from build123d import *

# Parameters (mm, degrees)
SKETCH1_R           = 5.715
BOSS_EXTRUDE1_DEPTH = 12.7
SKETCH2_R           = 1.4732
CUT_EXTRUDE1_DEPTH  = 16.053652381
SKETCH3_W           = 7
SKETCH3_H           = 6
BOSS_EXTRUDE2_DEPTH = 7


with BuildPart() as part:
    # Sketch1 → Boss-Extrude1 (new body)
    with BuildSketch(Plane.XY):
        with Locations(Location((0, 0, 0), (0, 0, 180))):
            Circle(SKETCH1_R)
    extrude(amount=BOSS_EXTRUDE1_DEPTH)

    # Sketch2 → Cut-Extrude1 (cut, through all)
    with BuildSketch(Plane.XY.offset(12.7)):
        Circle(SKETCH2_R)
    extrude(amount=-CUT_EXTRUDE1_DEPTH, mode=Mode.SUBTRACT)

    # Sketch3 → Boss-Extrude2 (add)
    with BuildSketch(Plane(origin=(4, 0, 0), x_dir=(0, 0, -1), z_dir=(1, 0, 0))):
        with Locations((-6.35, 0)):
            Rectangle(SKETCH3_W, SKETCH3_H)
    extrude(amount=BOSS_EXTRUDE2_DEPTH)


solid = part.part
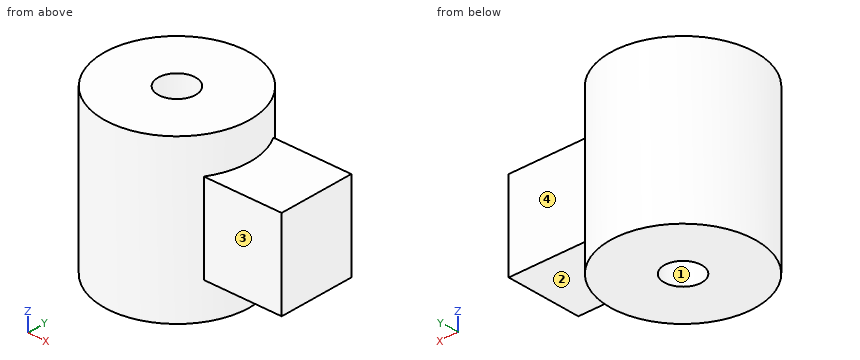
Read the model definition and answer for the solid it produces. Units are mm, in the model's axes. Face numbers are marked on the shaded views. Give positions to 0.01 mm unless a question says otherwise; leave off trailing zeros. Write each loop counter-clockwise with the first axis right and the second up, starting at its lowest first coordinate (ties: lowest second). Pieces come first, ordered by that corner, then holes. Notation, with made-up numbers: (-36, 11.5) -> (-13, 11.5) arc R30 cw to (-13, 40.5) -> close; hole circle Ø11 at (-29, 15). An arc over 180 degrees is marked (long way). Answer as a JSON object with one key per item and string values. Group by question number.
1) Consider L1, parallel to Y at x = 0, z = 5 (3 decimals); L2, parallel to Y at x = 7.25, z = 8; L3, parallel to Z at x = 9.5, y = -0.5. Determine where each line is inside the solid, lowest interval first. Write a range as from..to.
2) Each of these flat-tipped pins is pushed along its axis until it touches: P1, Ø4, axis at x = 7, z = 4.5, coming from the -Y side; P2, Ø6.5, axis at x = 8.5, z = 6, coming from the +Y side; P3, Ø3, axis at x = 8, y = -0.5, coming from the -Z side. Where does it stop, or does it pass through?
3) The mould has two halves that part along Y. Classify the marked faces 1, 2, 3 and 4: +Y half, -Y half, draft (parallel to the pull), parting line (faces both ways), or undercut.
4) Find section A-A (x = 0). Write down the section's boundary in (y, z) (3 decimals).
5) Find section D-D (y = 2.5). Write down the section's boundary in (x, z), and give its area (3 significant figures).
6) Find section C-C (z = 10.5). Write down the section's boundary in (x, y) (3 decimals).
7) Find section B-B (y = 0). Write down the section's boundary in (x, z) (3 decimals), and give its area (3 significant figures).
Values follow:
{
 "1": {"L1": "y = -5.715..-1.473, 1.473..5.715", "L2": "y = -3..3", "L3": "z = 2.85..9.85"},
 "2": {"P1": "stops at y = -3", "P2": "stops at y = 3", "P3": "stops at z = 2.85"},
 "3": {"face 1": "undercut", "face 2": "draft", "face 3": "-Y half", "face 4": "+Y half"},
 "4": {"outline": "(-5.715, 0) -> (-1.473, 0) -> (-1.473, 12.7) -> (-5.715, 12.7) -> close; (1.473, 0) -> (5.715, 0) -> (5.715, 12.7) -> (1.473, 12.7) -> close"},
 "5": {"outline": "(-5.14, 0) -> (5.14, 0) -> (5.14, 2.85) -> (11, 2.85) -> (11, 9.85) -> (5.14, 9.85) -> (5.14, 12.7) -> (-5.14, 12.7) -> close", "area": "172 mm2"},
 "6": {"outline": "circle Ø11.43 at (0, 0); hole circle Ø2.946 at (0, 0)"},
 "7": {"outline": "(-5.715, 0) -> (-1.473, 0) -> (-1.473, 12.7) -> (-5.715, 12.7) -> close; (1.473, 0) -> (5.715, 0) -> (5.715, 2.85) -> (11, 2.85) -> (11, 9.85) -> (5.715, 9.85) -> (5.715, 12.7) -> (1.473, 12.7) -> close", "area": "145 mm2"}
}
